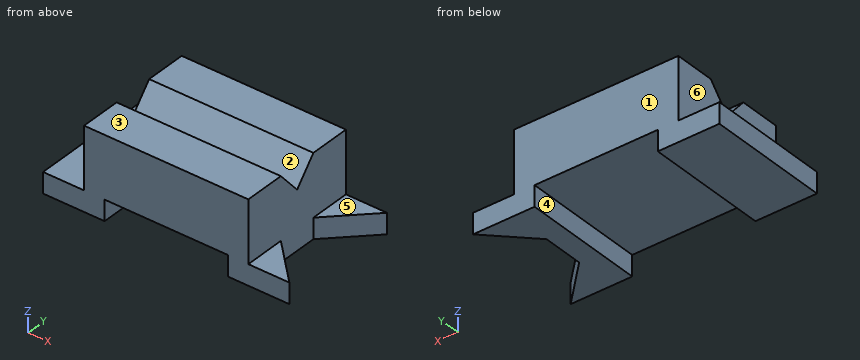
from build123d import *

# Parameters (mm, degrees)
F1_DEPTH = 76.2
F3_DEPTH = 152.4
F5_DEPTH = 12.7


with BuildPart() as f1:
    # F0 (on Front) → F1 (new body)
    with BuildSketch(Plane.XZ):
        Polygon((0, 12.7), (0, 0), (38.1, 0), (38.1, 12.7), (114.3, 12.7), (114.3, 0), (127, 0), (127, 50.8), (25.4, 50.8), (25.4, 12.7), align=None)
    extrude(amount=F1_DEPTH)

    # F2 (on face) → F3 (cut)
    with BuildSketch(Plane(origin=(25.4, 0, 0), x_dir=(0, -1, 0), z_dir=(-1, 0, 0))):
        Polygon((50.8, 50.8), (25.4, 50.8), (38.1, 35.975717), align=None)
    extrude(amount=-F3_DEPTH, mode=Mode.SUBTRACT)

    # F4 (on face) → F5 (join)
    with BuildSketch(Plane(origin=(0, 0, 0), x_dir=(1, 0, 0), z_dir=(0, 0, -1))):
        Polygon((152.4, 76.2), (127, 76.2), (127, 50.8), align=None)
        Polygon((127, 25.4), (127, 0), (152.4, 0), align=None)
    extrude(amount=-F5_DEPTH)


solid = f1.part
Read the model definition and answer for the solid it produces. Units are mm, in the model's axes. Face numbers are marked on the shaded views. A direction names the side the tool comes from. Give positions to 0.01 mm unless a question says otherwise; leave off trailing zeros. Loops run counter-clockwise (first coordinate to the right, second up) from the corner with the lowest first, then second, coordinate; pieces in that order, holes last. Notation, with made-up numbers: (13.5, 32.25) -> (66.5, 32.25) arc R24 ccw to (66.5, 55.25) -> close; hole circle Ø3 at (-24, -4). An arc over 180 degrees is marked (long way). Use a Markdown table: item, result.
Q1. Section D-D, the plane x = 120 is taken. Determine the outline of the cut face in (y, z).
Solved:
| item | result |
|---|---|
| outline | (-76.2, 0) -> (0, 0) -> (0, 50.8) -> (-25.4, 50.8) -> (-38.1, 35.98) -> (-50.8, 50.8) -> (-76.2, 50.8) -> close |
Q2. Section C-C, the plane y = -14 is taken. Determine the outline of the cut face in (x, z), then the cut area to 3 significant figures.
Solved:
| item | result |
|---|---|
| outline | (0, 0) -> (38.1, 0) -> (38.1, 12.7) -> (114.3, 12.7) -> (114.3, 0) -> (138.4, 0) -> (138.4, 12.7) -> (127, 12.7) -> (127, 50.8) -> (25.4, 50.8) -> (25.4, 12.7) -> (0, 12.7) -> close |
| area | 4,660 mm^2 |
Q3. Find the intervals of material crossed by line 1 along X through (y, z) = (-44.5, 2.5); line 2 along Z through (x, y) = (85, -70); line 3 along X through (y, z) = (-18.5, 43), in increasing order.
Solved:
| item | result |
|---|---|
| line 1 | x = 0 to 38.1, 114.3 to 127 |
| line 2 | z = 12.7 to 50.8 |
| line 3 | x = 25.4 to 127 |
Q4. Determine the mould class of the marked faces 1, 2 and 3 for opening direction Y: pulls with the +Y half, pulls with the -Y half, needs draft (parallel to the pull), parting line crosses it, or undercut.
Solved:
| item | result |
|---|---|
| face 1 | pulls with the +Y half |
| face 2 | undercut |
| face 3 | needs draft |
Q5. Section B-B, the plane z = 3 is taken. Determine the outline of the cut face in (x, y), then the cut area to 3 significant figures.
Solved:
| item | result |
|---|---|
| outline | (0, -76.2) -> (38.1, -76.2) -> (38.1, 0) -> (0, 0) -> close; (114.3, -76.2) -> (152.4, -76.2) -> (127, -50.8) -> (127, -25.4) -> (152.4, 0) -> (114.3, 0) -> close |
| area | 4,520 mm^2 |
Q6. Section A-A, the plane x = 141 is taken. Determine the outline of the cut face in (y, z).
Solved:
| item | result |
|---|---|
| outline | (-76.2, 0) -> (-64.8, 0) -> (-64.8, 12.7) -> (-76.2, 12.7) -> close; (-11.4, 0) -> (0, 0) -> (0, 12.7) -> (-11.4, 12.7) -> close |
Q7. A tool of negligible diameter and unlimited length cuts with its end or side. For the marked faces 4, 5 and 6, from which of +Z, -Z, +X, -X, +Y, -Y can it reach the whole face along a straight path? Write none if from no direction.
Solved:
| item | result |
|---|---|
| face 4 | -Z, +Y, -Y |
| face 5 | +Z, +X, +Y, -Y |
| face 6 | +Z, -X, +Y, -Y |
Q8. Each of these flat-tipped pins is pushed along its axis until it touches: pin 1 (2 mm diameter, centred on y = -43.5, z = 43, fed in from -X); pin 2 (12.5 mm diameter, centred on x = 137, y = -64.5, fed in from +Z); pin 3 (2 mm diameter, centred on x = 51, y = -32, fed in from +Z). Where does it stop, or does it pass through?
Solved:
| item | result |
|---|---|
| pin 1 | stops at x = 25.4 |
| pin 2 | stops at z = 12.7 |
| pin 3 | stops at z = 44.26 |
